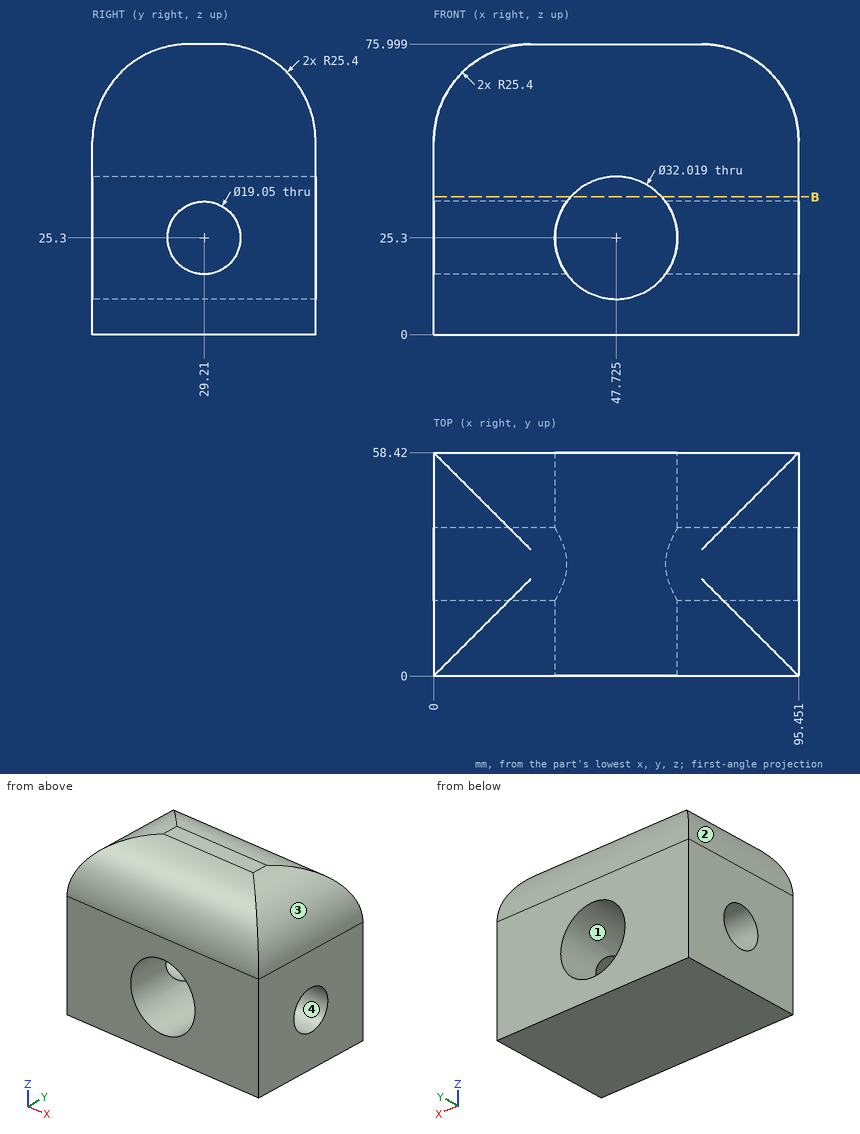
Part print with two shaded views. Sizes in mm from the minimum x, y, z corner. Round coordinates to 2 decimals unless told otherwise and drop trailing zeros. Order: outer loops, then holes, each group sorted by start corner. A loop starts at its lowest first (then second) coordinate and runs counter-clockwise, first axis right, second up.
(1) Pin check, flat tips, straight feed: pin 1 (12 mm diameter, centred on x = 16.5, z = 60.5, fed in from +Y); pin 2 (2 mm diameter, centred on x = 39.5, y = 49.5, fed in from +Z); pin 3 (4 mm diameter, centred on x = 53.5, z = 60.5, fed in from -Y). Stop position of each tip, or through.
(2) Drill centre lines: line 1 (Z direction, x = 81, y = 29.21) (1 decimal); line 2 (Z direction, x = 40.5, y = 45) (1 decimal); line 3 (X direction, y = 31.5, z = 52). Where is each one in solid material? Low to high.
(3) Pull direction X, two halves, no side cores. Call the marked faces 1, 2, 3 and 4: released by +X, released by -X, zero draft, split by the parting line, or undercut.
(4) Band-saw the part on B-B (z = 36). List the corners of the cut face in (x, y).
Verdict:
1. pin 1: stops at y = 58.12
1. pin 2: stops at z = 70.74
1. pin 3: stops at y = 1.26
2. line 1: z = 0 to 15.8, 34.8 to 73.5
2. line 2: z = 0 to 11, 39.6 to 73
2. line 3: x = 0.04 to 95.41
3. face 1: undercut
3. face 2: released by -X
3. face 3: released by +X
3. face 4: zero draft
4. outline: (0, 0) - (35.82, 0) - (35.82, 58.42) - (0, 58.42) - close; (59.63, 0) - (95.45, 0) - (95.45, 58.42) - (59.63, 58.42) - close
